Could you check a few things on this model? Use its own coordinates, in mm. A direction names the side the tool comes from. Round coordinates to 2 decimals unless told otherwise and drop trailing zeros. Loops run counter-clockwise (first coordinate to the right, second up) from the corner with the lowest first, then second, coordinate; pieces in that order, holes last.
from build123d import *

# Parameters (mm, degrees)
F1_DEPTH = 1.75
F3_DEPTH = 9
F4_SIZE  = 4


with BuildPart() as f1:
    # F0 (on Front) → F1 (new body)
    with BuildSketch(Plane.XZ):
        Polygon((0, 690), (-280, 543.521333), (-280, -146.478667), (0, 0), align=None)
    extrude(amount=F1_DEPTH)

    # F2 (on face) → F3 (join)
    with BuildSketch(Plane.XZ.offset(1.75)):
        Polygon((-120.85038, 612.445705), (-196.166836, 573.044798), (-168.35443, 519.880241), (-93.037975, 559.281148), align=None)
    extrude(amount=F3_DEPTH)

    # F4
    f4_edges = [f1.edges().sort_by_distance(p)[0] for p in [
        (-106.944177, -10.75, 585.863427),
        (-158.508608, -10.75, 592.745251),
        (-182.260633, -10.75, 546.462519),
        (-130.696203, -10.75, 539.580694),
    ]]
    chamfer(f4_edges, length=F4_SIZE)


solid = f1.part
Item 1: If I drill on line 1 along Y through (x, z) = (-251, -77); line 2 along Z through (x, y) = (-125.5, -1.5); line 3 along Z through (x, y) = (-174, -7), over which ranges is the centre line in solid material (lowest first)?
Results list:
line 1: y = -1.75 to 0
line 2: z = -65.65 to 624.35
line 3: z = 531.21 to 584.36
Item 2: For faces 1 (the flat face through (-157.98, -4.22, 593.02)), 2 (the flat face through (-131.223, -4.215, 539.305)), 3 (the flat face through (-106.75, -4.22, 585.49)), which set-ups out of +Z, -Z, +X, -X, +Y, -Y let a thin tool reach every point of the face, with its end or its side?
Results list:
face 1: +Z, -X, -Y
face 2: -Z, +X, -Y
face 3: +Z, +X, -Y
Item 3: If we section it at B-B, the plane x = -150.5: Please give me the cut outline in (y, z).
Results list:
outline: (-10.75, 533.73) - (-6.75, 529.22) - (-1.75, 529.22) - (-1.75, -78.73) - (0, -78.73) - (0, 611.27) - (-1.75, 611.27) - (-1.75, 596.93) - (-6.75, 596.93) - (-10.75, 592.42) - close
Item 4: If we section it at D-D, the plane z = 301: Please give me the cut outline in (x, y), then the cut area to 3 significant figures.
Results list:
outline: (-280, -1.75) - (0, -1.75) - (0, 0) - (-280, 0) - close
area: 490 mm2
Item 5: Will this pin go through, and if not, where does the flat tip stop? pin 1 (6 mm diameter, centred on x = -164.5, y = -5.5, fed in from +Z).
Results list:
pin 1: stops at z = 591.18
Item 6: If we section it at C-C, the plane y = -9: Please give me the cut outline in (x, z), then the cut area to 3 significant figures.
Results list:
outline: (-193.13, 572.09) - (-167.4, 522.92) - (-96.07, 560.23) - (-121.8, 609.41) - close
area: 4,470 mm2
Item 7: If we section it at A-A, the plane z = 597: Please give me the cut outline in (x, y).
Results list:
outline: (-177.77, -1.75) - (-150.38, -1.75) - (-150.38, -6.75) - (-141.75, -10.75) - (-117.28, -10.75) - (-112.77, -6.75) - (-112.77, -1.75) - (0, -1.75) - (0, 0) - (-177.77, 0) - close
